For this review, take the finished solid that the model builds, in its own axes (mm). Give positions to 0.01 mm unless a question says otherwise; leave off trailing zeros. Order: outer loops, then holes, each group sorted by start corner. A loop starts at its lowest first (then second) coordinate and runs counter-clockwise, first axis right, second up. Notation, with made-up numbers: (70.25, 24.5) - (117.25, 24.5) arc R20 cw to (117.25, 45.5) - close; hole circle Ø4 at (-30.75, -30). An arc over 180 degrees is marked (long way). One line per item, written item: value.
```python
from build123d import *

# Parameters (mm, degrees)
SKETCH_1_W      = 40
SKETCH_1_H      = 100
SKETCH_1_R      = 2.1
EXTRUDE_1_DEPTH = 3
FILLET_1_R      = 3


with BuildPart() as part:
    # ｽｹｯﾁ1 → ﾎﾞｽ - 押し出し1 (new body)
    with BuildSketch(Plane(origin=(0, 0, 0), x_dir=(1, 0, 0), z_dir=(0, 1, 0))):
        Rectangle(SKETCH_1_W, SKETCH_1_H)
        with Locations(Location((14.25, 23.75, 0), (0, 0, 270))):
            Circle(SKETCH_1_R, mode=Mode.SUBTRACT)
        with Locations(Location((-14.25, 23.75, 0), (0, 0, 90))):
            Circle(SKETCH_1_R, mode=Mode.SUBTRACT)
        with Locations(Location((-14.25, -23.75, 0), (0, 0, 270))):
            Circle(SKETCH_1_R, mode=Mode.SUBTRACT)
        with Locations(Location((14.25, -23.75, 0), (0, 0, 90))):
            Circle(SKETCH_1_R, mode=Mode.SUBTRACT)
        with Locations(Location((7.5, 45, 0), (0, 0, 270))):
            Circle(SKETCH_1_R, mode=Mode.SUBTRACT)
        with Locations(Location((-7.5, 45, 0), (0, 0, 90))):
            Circle(SKETCH_1_R, mode=Mode.SUBTRACT)
        with Locations(Location((-7.5, -45, 0), (0, 0, 270))):
            Circle(SKETCH_1_R, mode=Mode.SUBTRACT)
        with Locations(Location((7.5, -45, 0), (0, 0, 90))):
            Circle(SKETCH_1_R, mode=Mode.SUBTRACT)
        with Locations(Location((0, 23.75, 0), (0, 0, 270))):
            Circle(SKETCH_1_R, mode=Mode.SUBTRACT)
        with Locations(Location((0, -23.75, 0), (0, 0, 90))):
            Circle(SKETCH_1_R, mode=Mode.SUBTRACT)
    extrude(amount=EXTRUDE_1_DEPTH)

    # ﾌｨﾚｯﾄ1
    fillet_1_edges = [part.edges().sort_by_distance(p)[0] for p in [
        (20, 1.5, 50),
        (-20, 1.5, 50),
        (-20, 1.5, -50),
        (20, 1.5, -50),
    ]]
    fillet(fillet_1_edges, radius=FILLET_1_R)


solid = part.part
```
(1) Take a section at A-A (z = 23.75). Write out the cut boundary in (x, y).
Answers below:
outline: (-20, 0) - (-16.35, 0) - (-16.35, 3) - (-20, 3) - close; (-12.15, 0) - (-2.1, 0) - (-2.1, 3) - (-12.15, 3) - close; (2.1, 0) - (12.15, 0) - (12.15, 3) - (2.1, 3) - close; (16.35, 0) - (20, 0) - (20, 3) - (16.35, 3) - close
(2) Take a section at C-C (y = 1.35). Give the number of separate pieces and of enclosed holes in the cut face, then the cut area to 3 significant figures.
Answers below:
separate pieces: 1
enclosed holes: 10
area: 3,850 mm^2
(3) Take a section at B-B (x = 7.5). Write out the cut boundary in (y, z).
Answers below:
outline: (0, -50) - (3, -50) - (3, -47.1) - (0, -47.1) - close; (0, -42.9) - (3, -42.9) - (3, 42.9) - (0, 42.9) - close; (0, 47.1) - (3, 47.1) - (3, 50) - (0, 50) - close
(4) Wall thickness on line 1 (X direction, y = 1.6, z = 23.75); line 2 (X direction, y = 2.2, z = 45); line 3 (Z direction, x = -8, y = 0.65): over which ranges is each line inside the solid? List them lowest first. Write a range as from..to.
Answers below:
line 1: x = -20..-16.35, -12.15..-2.1, 2.1..12.15, 16.35..20
line 2: x = -20..-9.6, -5.4..5.4, 9.6..20
line 3: z = -50..-47.04, -42.96..42.96, 47.04..50
(5) Take a section at D-D (z = -45). Write out the cut boundary in (x, y), then the cut area to 3 significant figures.
Answers below:
outline: (-20, 0) - (-9.6, 0) - (-9.6, 3) - (-20, 3) - close; (-5.4, 0) - (5.4, 0) - (5.4, 3) - (-5.4, 3) - close; (9.6, 0) - (20, 0) - (20, 3) - (9.6, 3) - close
area: 94.8 mm^2
(6) Draft analysis for pull direction X (two halves, no side actions). For faces 1 (the face through (-0.8, 1.48, -21.81)), 2 (the face through (0, 3, -1)), 3 (the face through (20, 1, 1)), 4 (the face through (-19.14, 1.52, 49.1)), state which applies: pulls with the +X half, pulls with the -X half, needs draft (parallel to the pull), parting line crosses it, or undercut.
Answers below:
face 1: undercut
face 2: needs draft
face 3: pulls with the +X half
face 4: pulls with the -X half
